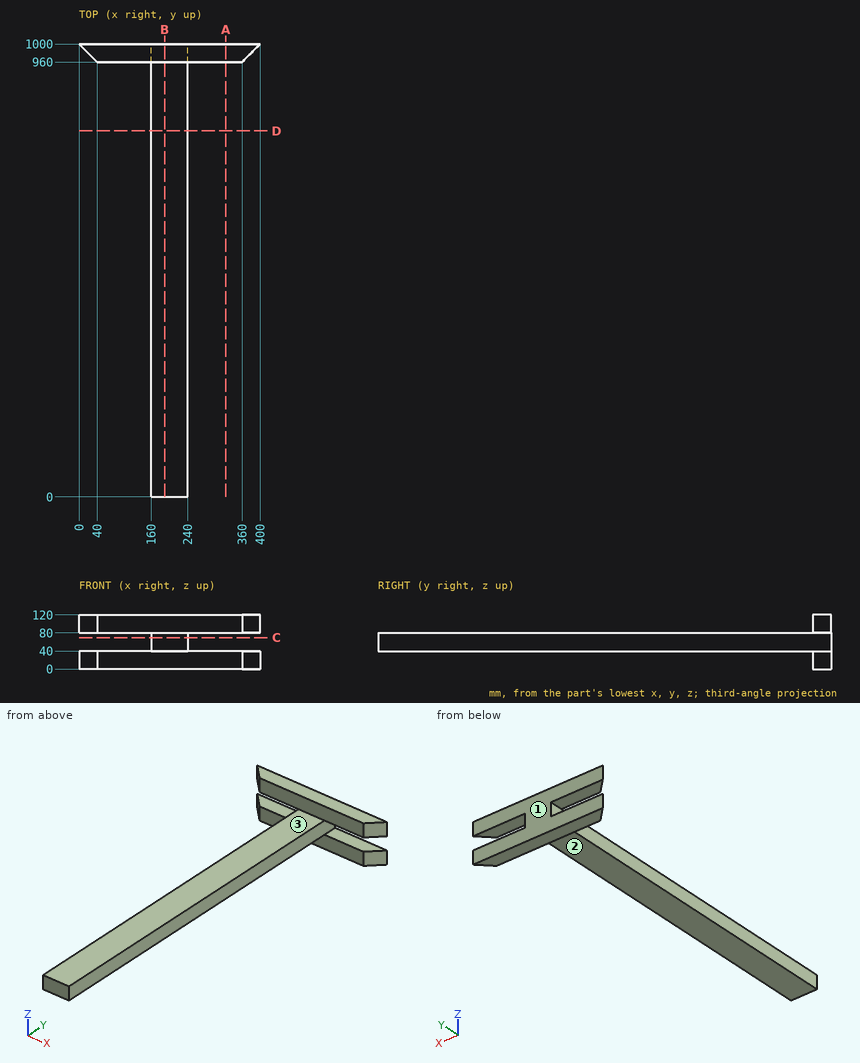
Geometry check sheet. Reference: drawing and pictorial views, mm from the part's lowest x, y, z. A direction names the side the tool comes from. Round coordinates to 2 decimals unless told otherwise and drop trailing zeros. Loops run counter-clockwise (first coordinate to the right, second up) from the corner with the lowest first, then second, coordinate; pieces in that order, holes last. Notation, with made-up numbers: (-13, 44.25) - (-9, 44.25) arc R18 cw to (-9, 59.25) - close; hole circle Ø10 at (-3.75, 89.25). An arc over 180 degrees is marked (long way). Use a Markdown table: item, result. Add a question column.
1. Gauge pin test, flat ends, axial feed: pin 1 (12 mm diameter, centred on x = 117, z = 72.5, fed in from +Y); pin 2 (8 mm diameter, centred on x = 219.5, z = 23.5, fed in from -Y); pin 3 (20 mm diameter, centred on y = 502.5, z = 53.5, fed in from +X); pin 4 (4 mm diameter, centred on y = 491.5, z = 73.5, fed in from -X). Record the tip position at first contact, or that the pin passes through.
2. Section check B-B, the plane x = 189. Record the boundary of the cut face in (y, z), plus the area to 3 significant figures.
3. Thickness scan on probe 1 along Y at (x, z) = (242.5, 22); probe 2 along X at (y, z) = (331, 58); probe 3 along Z at (x, y) = (173, 648.5). Record the ranges inside material, lowest first. Write a range as [from, to].
4. Section check A-A, the plane x = 324.5. Record the boundary of the cut face in (y, z), plus the area to 3 significant figures.
5. Section check C-C, the plane z = 69.5. Record the boundary of the cut face in (x, y).
6. Section check D-D, the plane y = 808. Record the boundary of the cut face in (x, z), plus the area to 3 significant figures.
7. Access from +Z, -Z, +X, -X, +Y, -Y to the whole of each face (thin tool, end or side, straight path). Record for the marked faces 1, 2 and 3.
Checks:
| question | item | result |
|---|---|---|
| 1 | pin 1 | passes through |
| 1 | pin 2 | stops at y = 960 |
| 1 | pin 3 | stops at x = 240 |
| 1 | pin 4 | stops at x = 160 |
| 2 | outline | (0, 40) - (960, 40) - (960, 0) - (1000, 0) - (1000, 120) - (960, 120) - (960, 80) - (0, 80) - close |
| 2 | area | 43,200 mm^2 |
| 3 | probe 1 | y = [960, 1000] |
| 3 | probe 2 | x = [160, 240] |
| 3 | probe 3 | z = [40, 80] |
| 4 | outline | (960, 0) - (1000, 0) - (1000, 40) - (960, 40) - close; (960, 80) - (1000, 80) - (1000, 120) - (960, 120) - close |
| 4 | area | 3,200 mm^2 |
| 5 | outline | (160, 0) - (240, 0) - (240, 1000) - (160, 1000) - close |
| 6 | outline | (160, 40) - (240, 40) - (240, 80) - (160, 80) - close |
| 6 | area | 3,200 mm^2 |
| 7 | face 1 | +Z, -Z, +X, -X, +Y |
| 7 | face 2 | -Z, +X, -X, -Y |
| 7 | face 3 | +Z, +X, -X, -Y |
